CAD build for the part. Positions are in the model's coordinates, mm. A direction names the side the tool comes from. Give positions to 0.01 mm unless a question says otherwise; leave off trailing zeros. Write each loop counter-clockwise with the first axis right and the second up, starting at its lowest first coordinate (ties: lowest second). Pieces come first, ordered by that corner, then holes. Notation, with made-up numbers: (89.5, 8) - (144.5, 8) arc R23 cw to (144.5, 38) - close; hole circle Ø3 at (-21, -20). An arc over 180 degrees is marked (long way). Answer as a JSON object with one key per item and string values.
from build123d import *

# Parameters (mm, degrees)
SKETCH_1_W          = 45
SKETCH_1_H          = 45
EXTRUDE_1_DEPTH     = 8
SKETCH_2_R          = 2.75
CUT_EXTRUDE_1_DEPTH = 8
SKETCH_3_R          = 3.25
CUT_EXTRUDE_2_DEPTH = 8
SKETCH_4_R          = 7
CUT_EXTRUDE_3_DEPTH = 3


with BuildPart() as part:
    # 草图1 → 凸台-拉伸1 (new body)
    with BuildSketch(Plane(origin=(0, 0, 0), x_dir=(1, 0, 0), z_dir=(0, 1, 0))):
        Rectangle(SKETCH_1_W, SKETCH_1_H)
    extrude(amount=EXTRUDE_1_DEPTH)

    # 草图2 → 切除-拉伸1 (cut)
    with BuildSketch(Plane(origin=(0, 8, 0), x_dir=(1, 0, 0), z_dir=(0, 1, 0))):
        with Locations(Location((-16.25, 15, 0), (0, 0, 270))):
            Circle(SKETCH_2_R)
        with Locations(Location((16.25, 15, 0), (0, 0, 270))):
            Circle(SKETCH_2_R)
        with Locations(Location((16.25, -15, 0), (0, 0, 270))):
            Circle(SKETCH_2_R)
        with Locations(Location((-16.25, -15, 0), (0, 0, 270))):
            Circle(SKETCH_2_R)
    extrude(amount=-CUT_EXTRUDE_1_DEPTH, mode=Mode.SUBTRACT)

    # 草图3 → 切除-拉伸2 (cut)
    with BuildSketch(Plane(origin=(0, 8, 0), x_dir=(1, 0, 0), z_dir=(0, 1, 0))):
        with Locations(Location((0, 0, 0), (0, 0, 270))):
            Circle(SKETCH_3_R)
    extrude(amount=-CUT_EXTRUDE_2_DEPTH, mode=Mode.SUBTRACT)

    # 草图4 → 切除-拉伸3 (cut)
    with BuildSketch(Plane.XZ):
        with Locations(Location((0, 0, 0), (0, 0, 270))):
            Circle(SKETCH_4_R)
    extrude(amount=-CUT_EXTRUDE_3_DEPTH, mode=Mode.SUBTRACT)


solid = part.part
(1) Saw through at B-B, the plane x = 0. Give the cut face in (y, z), and give its area (4 significant figures).
Answer key:
{"outline": "(0, -22.5) - (8, -22.5) - (8, -3.25) - (3, -3.25) - (3, -7) - (0, -7) - close; (0, 7) - (3, 7) - (3, 3.25) - (8, 3.25) - (8, 22.5) - (0, 22.5) - close", "area": "285.5 mm²"}
(2) Saw through at C-C, the plane y = 5.5. Give the cut face in (x, z), and give its area (3 significant figures).
Answer key:
{"outline": "(-22.5, -22.5) - (22.5, -22.5) - (22.5, 22.5) - (-22.5, 22.5) - close; hole circle Ø5.5 at (-16.25, -15); hole circle Ø5.5 at (-16.25, 15); hole circle Ø6.5 at (0, 0); hole circle Ø5.5 at (16.25, -15); hole circle Ø5.5 at (16.25, 15)", "area": "1,900 mm²"}
(3) Flat gauge pins, fed straight in: P1, Ø12, axis at x = 2, z = 11, coming from the -Y side; P2, Ø4, axis at x = -1, z = 0, coming from the -Y side. Where does each tip first touch, or does it go through?
Answer key:
{"P1": "stops at y = 0", "P2": "passes through"}
(4) 3-axis set-ups, long thin cutter, end or side, ignore diameter. For faces 4 (the face through (0, 8, -5)), 5 (the face through (2, 3, -3)): which of +Z, -Z, +X, -X, +Y, -Y reach the whole face in a straight line?
Answer key:
{"face 4": "+Z, -Z, +X, -X, +Y", "face 5": "-Y"}
(5) Probe L1, parallel to X at y = 2.75, z = 15; L2, parallel to Z at x = -15, y = 4; L3, parallel to X at y = 5.95, z = 0. List the from-to ranges inside material, lowest first. Write a range as [from, to].
Answer key:
{"L1": "x = [-22.5, -19], [-13.5, 13.5], [19, 22.5]", "L2": "z = [-22.5, -17.45], [-12.55, 12.55], [17.45, 22.5]", "L3": "x = [-22.5, -3.25], [3.25, 22.5]"}
(6) Pull direction Z, two halves, no side cores. Call faces 1 (the face through (-22.5, 4, 0)), 2 (the face through (16.371, 4.056, -17.747)), 3 (the face through (0, 4, 22.5)): pulls with the +Z half, pulls with the -Z half, needs draft (parallel to the pull), parting line crosses it, or undercut.
Answer key:
{"face 1": "needs draft", "face 2": "undercut", "face 3": "pulls with the +Z half"}
(7) Saw through at A-A, the plane z = 0. Give the cut face in (x, y), and give its area (4 significant figures).
Answer key:
{"outline": "(-22.5, 0) - (-7, 0) - (-7, 3) - (-3.25, 3) - (-3.25, 8) - (-22.5, 8) - close; (3.25, 3) - (7, 3) - (7, 0) - (22.5, 0) - (22.5, 8) - (3.25, 8) - close", "area": "285.5 mm²"}
(8) Saw through at D-D, the plane x = 16.25. Give the cut face in (y, z), and give its area (3 significant figures).
Answer key:
{"outline": "(0, -22.5) - (8, -22.5) - (8, -17.75) - (0, -17.75) - close; (0, -12.25) - (8, -12.25) - (8, 12.25) - (0, 12.25) - close; (0, 17.75) - (8, 17.75) - (8, 22.5) - (0, 22.5) - close", "area": "272 mm²"}
